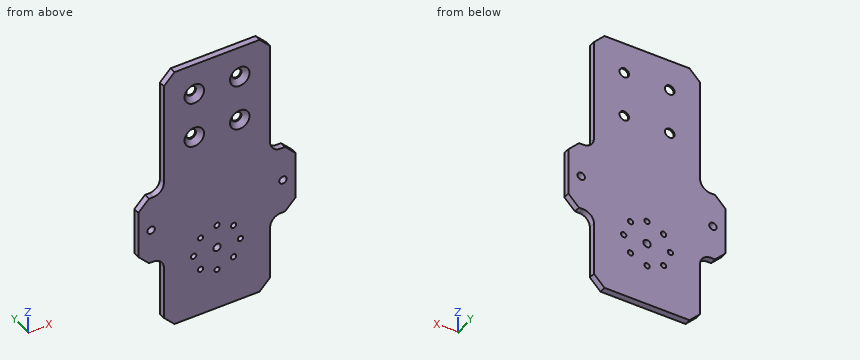
from build123d import *

# Parameters (mm, degrees)
SKETCH1_W                                    = 50
SKETCH1_H                                    = 125
BOSS_EXTRUDE1_DEPTH                          = 3
SKETCH2_R                                    = 1.75
CUT_EXTRUDE1_DEPTH                           = 10
SKETCH14_R                                   = 2
CUT_EXTRUDE16_DEPTH                          = 10
CSK_FOR_M4_HEX_SOCKET_COUNTERSUNK_HE_2_COUNT = 2
CSK_FOR_M4_HEX_SOCKET_COUNTERSUNK_HE_2_PITCH = 21.4
CSK_FOR_M4_HEX_SOCKET_COUNTERSUNK_HE_3_COUNT = 2
CSK_FOR_M4_HEX_SOCKET_COUNTERSUNK_HE_3_PITCH = 30.264170235
CSK_FOR_M4_HEX_SOCKET_COUNTERSUNK_HE_4_COUNT = 2
CSK_FOR_M4_HEX_SOCKET_COUNTERSUNK_HE_4_PITCH = 21.4
CUT_EXTRUDE17_REACH                          = 69.381
SKETCH18_R                                   = 1.25
CHAMFER1_SIZE                                = 5
SKETCH19_W                                   = 12
SKETCH19_H                                   = 32
BOSS_EXTRUDE2_DEPTH                          = 3
CHAMFER2_SIZE                                = 5
FILLET1_R                                    = 5
SKETCH20_R                                   = 1.75
CUT_EXTRUDE18_DEPTH                          = 73.692846966


with BuildPart() as part:
    # Sketch1 → Boss-Extrude1 (new body)
    with BuildSketch(Plane(origin=(0, 0, 0), x_dir=(1, 0, 0), z_dir=(0, 1, 0))):
        Rectangle(SKETCH1_W, SKETCH1_H)
    extrude(amount=BOSS_EXTRUDE1_DEPTH)

    # Sketch2 → Cut-Extrude1 (cut)
    with BuildSketch(Plane(origin=(0, 3, 0), x_dir=(1, 0, 0), z_dir=(0, 1, 0))):
        with Locations(Location((0, 32.5, 0), (0, 0, 270))):
            Circle(SKETCH2_R)
    extrude(amount=-CUT_EXTRUDE1_DEPTH, mode=Mode.SUBTRACT)

    # Sketch14 → Cut-Extrude16 (cut)
    with BuildSketch(Plane(origin=(0, 3, 0), x_dir=(1, 0, 0), z_dir=(0, 1, 0))):
        with Locations(Location((-10.7, -26.6, 0), (0, 0, 270))):
            Circle(SKETCH14_R)
        with Locations(Location((10.7, -26.6, 0), (0, 0, 270))):
            Circle(SKETCH14_R)
        with Locations(Location((10.7, -48, 0), (0, 0, 270))):
            Circle(SKETCH14_R)
        with Locations(Location((-10.7, -48, 0), (0, 0, 270))):
            Circle(SKETCH14_R)
    extrude(amount=-CUT_EXTRUDE16_DEPTH, mode=Mode.SUBTRACT)

    # Sketch15 → CSK for M4 Hex Socket Countersunk Head Screw1 (revolve, cut)
    with BuildSketch(Plane(origin=(-10.7, 0, 26.6), x_dir=(0, 0, -1), z_dir=(1, 0, 0))):
        Polygon((0, 0), (0, 3), (2.25, 3), (2.25, 2.34), (4.59, 0), align=None)
    csk_for_m4_hex_socket_countersunk_head_s = revolve(axis=Axis((-10.7, -6.35, 26.6), (0, 1, 0)), mode=Mode.SUBTRACT)

    # CSK for M4 Hex Socket Countersunk He 2: CSK for M4 Hex Socket Countersunk Head Screw1 ×2
    with Locations(*[(i * CSK_FOR_M4_HEX_SOCKET_COUNTERSUNK_HE_2_PITCH, 0, 0) for i in range(1, CSK_FOR_M4_HEX_SOCKET_COUNTERSUNK_HE_2_COUNT)]):
        add(csk_for_m4_hex_socket_countersunk_head_s, mode=Mode.SUBTRACT)

    # CSK for M4 Hex Socket Countersunk He 3: CSK for M4 Hex Socket Countersunk Head Screw1 ×2
    with Locations(*[Vector(0.7071067811865474, 0, 0.7071067811865477) * (i * CSK_FOR_M4_HEX_SOCKET_COUNTERSUNK_HE_3_PITCH) for i in range(1, CSK_FOR_M4_HEX_SOCKET_COUNTERSUNK_HE_3_COUNT)]):
        add(csk_for_m4_hex_socket_countersunk_head_s, mode=Mode.SUBTRACT)

    # CSK for M4 Hex Socket Countersunk He 4: CSK for M4 Hex Socket Countersunk Head Screw1 ×2
    with Locations(*[(0, 0, i * CSK_FOR_M4_HEX_SOCKET_COUNTERSUNK_HE_4_PITCH) for i in range(1, CSK_FOR_M4_HEX_SOCKET_COUNTERSUNK_HE_4_COUNT)]):
        add(csk_for_m4_hex_socket_countersunk_head_s, mode=Mode.SUBTRACT)

    # Sketch18 → Cut-Extrude17 (cut, up to next)
    with BuildSketch(Plane.XZ, mode=Mode.PRIVATE) as cut_extrude17_sk1:
        with Locations(Location((0, -21.5, 0), (0, 0, 270))):
            Circle(SKETCH18_R)
    cut_extrude17_tool1 = extrude(cut_extrude17_sk1.sketch, amount=-CUT_EXTRUDE17_REACH, mode=Mode.PRIVATE) & part.part
    # Sketch18 → Cut-Extrude17 (cut, up to next)
    with BuildSketch(Plane.XZ, mode=Mode.PRIVATE) as cut_extrude17_sk2:
        with Locations(Location((0, -43.5, 0), (0, 0, 270))):
            Circle(SKETCH18_R)
    cut_extrude17_tool2 = extrude(cut_extrude17_sk2.sketch, amount=-CUT_EXTRUDE17_REACH, mode=Mode.PRIVATE) & part.part
    # Sketch18 → Cut-Extrude17 (cut, up to next)
    with BuildSketch(Plane.XZ, mode=Mode.PRIVATE) as cut_extrude17_sk3:
        with Locations(Location((-11, -32.5, 0), (0, 0, 270))):
            Circle(SKETCH18_R)
    cut_extrude17_tool3 = extrude(cut_extrude17_sk3.sketch, amount=-CUT_EXTRUDE17_REACH, mode=Mode.PRIVATE) & part.part
    # Sketch18 → Cut-Extrude17 (cut, up to next)
    with BuildSketch(Plane.XZ, mode=Mode.PRIVATE) as cut_extrude17_sk4:
        with Locations(Location((11, -32.5, 0), (0, 0, 270))):
            Circle(SKETCH18_R)
    cut_extrude17_tool4 = extrude(cut_extrude17_sk4.sketch, amount=-CUT_EXTRUDE17_REACH, mode=Mode.PRIVATE) & part.part
    # Sketch18 → Cut-Extrude17 (cut, up to next)
    with BuildSketch(Plane.XZ, mode=Mode.PRIVATE) as cut_extrude17_sk5:
        with Locations(Location((7.778174593, -24.721825407, 0), (0, 0, 270))):
            Circle(SKETCH18_R)
    cut_extrude17_tool5 = extrude(cut_extrude17_sk5.sketch, amount=-CUT_EXTRUDE17_REACH, mode=Mode.PRIVATE) & part.part
    # Sketch18 → Cut-Extrude17 (cut, up to next)
    with BuildSketch(Plane.XZ, mode=Mode.PRIVATE) as cut_extrude17_sk6:
        with Locations(Location((-7.778174593, -24.721825407, 0), (0, 0, 270))):
            Circle(SKETCH18_R)
    cut_extrude17_tool6 = extrude(cut_extrude17_sk6.sketch, amount=-CUT_EXTRUDE17_REACH, mode=Mode.PRIVATE) & part.part
    # Sketch18 → Cut-Extrude17 (cut, up to next)
    with BuildSketch(Plane.XZ, mode=Mode.PRIVATE) as cut_extrude17_sk7:
        with Locations(Location((-7.778174593, -40.278174593, 0), (0, 0, 270))):
            Circle(SKETCH18_R)
    cut_extrude17_tool7 = extrude(cut_extrude17_sk7.sketch, amount=-CUT_EXTRUDE17_REACH, mode=Mode.PRIVATE) & part.part
    # Sketch18 → Cut-Extrude17 (cut, up to next)
    with BuildSketch(Plane.XZ, mode=Mode.PRIVATE) as cut_extrude17_sk8:
        with Locations(Location((7.778174593, -40.278174593, 0), (0, 0, 270))):
            Circle(SKETCH18_R)
    cut_extrude17_tool8 = extrude(cut_extrude17_sk8.sketch, amount=-CUT_EXTRUDE17_REACH, mode=Mode.PRIVATE) & part.part
    add(cut_extrude17_tool1.solids().sort_by_distance((0, 0, -21.5))[0], mode=Mode.SUBTRACT)
    add(cut_extrude17_tool2.solids().sort_by_distance((0, 0, -43.5))[0], mode=Mode.SUBTRACT)
    add(cut_extrude17_tool3.solids().sort_by_distance((-11, 0, -32.5))[0], mode=Mode.SUBTRACT)
    add(cut_extrude17_tool4.solids().sort_by_distance((11, 0, -32.5))[0], mode=Mode.SUBTRACT)
    add(cut_extrude17_tool5.solids().sort_by_distance((7.778175, 0, -24.721825))[0], mode=Mode.SUBTRACT)
    add(cut_extrude17_tool6.solids().sort_by_distance((-7.778175, 0, -24.721825))[0], mode=Mode.SUBTRACT)
    add(cut_extrude17_tool7.solids().sort_by_distance((-7.778175, 0, -40.278175))[0], mode=Mode.SUBTRACT)
    add(cut_extrude17_tool8.solids().sort_by_distance((7.778175, 0, -40.278175))[0], mode=Mode.SUBTRACT)

    # Chamfer1
    chamfer1_edges = [part.edges().sort_by_distance(p)[0] for p in [
        (-25, 1.5, -62.5),
        (25, 1.5, -62.5),
        (25, 1.5, 62.5),
        (-25, 1.5, 62.5),
    ]]
    chamfer(chamfer1_edges, length=CHAMFER1_SIZE)

    # Sketch19 → Boss-Extrude2 (add)
    with BuildSketch(Plane(origin=(0, 3, 0), x_dir=(1, 0, 0), z_dir=(0, 1, 0))):
        with Locations((-31, 11.5)):
            Rectangle(SKETCH19_W, SKETCH19_H)
        with Locations((31, 11.5)):
            Rectangle(SKETCH19_W, SKETCH19_H)
    extrude(amount=-BOSS_EXTRUDE2_DEPTH)

    # Chamfer2
    chamfer2_edges = [part.edges().sort_by_distance(p)[0] for p in [
        (37, 1.5, -27.5),
        (37, 1.5, 4.5),
        (-37, 1.5, -27.5),
        (-37, 1.5, 4.5),
    ]]
    chamfer(chamfer2_edges, length=CHAMFER2_SIZE)

    # Fillet1
    fillet1_edges = [part.edges().sort_by_distance(p)[0] for p in [
        (-25, 1.5, -27.5),
        (-25, 1.5, 4.5),
        (25, 1.5, -27.5),
        (25, 1.5, 4.5),
    ]]
    fillet(fillet1_edges, radius=FILLET1_R)

    # Sketch20 → Cut-Extrude18 (cut, through all)
    with BuildSketch(Plane(origin=(0, 3, 0), x_dir=(1, 0, 0), z_dir=(0, 1, 0))):
        with Locations(Location((-31, 11.5, 0), (0, 0, 270))):
            Circle(SKETCH20_R)
        with Locations(Location((31, 11.5, 0), (0, 0, 90))):
            Circle(SKETCH20_R)
    extrude(amount=-CUT_EXTRUDE18_DEPTH, mode=Mode.SUBTRACT)


solid = part.part
Check sheet for the modelled part. Datum: model origin and axes. Units: mm. Coordinates: 2 decimals unless noted, no trailing zeros. Write each loop counter-clockwise with the first axis right and the second up, starting at its lowest first coordinate (ties: lowest second). Pieces come first, ordered by that corner, then holes. Notation, with made-up numbers: M 56,74.5 L 115,74.5 A9 cw 115,87.5 Z; hole C 15,-16.75 d7. An arc over 180 degrees is marked long. Answer as CSV lines item,"result".
Q1. Cross-section at C-C (z = -43.5). Record the boundary of the cut face in (x, y).
Check result:
outline,"M -25,0 L -1.25,0 L -1.25,3 L -25,3 Z; M 1.25,0 L 25,0 L 25,3 L 1.25,3 Z"
Q2. Cross-section at D-D (y = 1.85). Count the separate pieces of the cut face and the enclosed holes in it, then the cut area to 3 significant figures.
Check result:
separate pieces,"1"
enclosed holes,"15"
area,"6,780 mm^2"
Q3. Material ranges on probe 1 along X at (y, z) = (2.8, 48); probe 2 along X at (y, z) = (0.25, -24); probe 3 along X at (y, z) = (1.65, -43.5), recorded low to high. Write a range as from..to.
Check result:
probe 1,"-25..-12.95, -8.45..8.45, 12.95..25"
probe 2,"-35.5..-8.8, -6.76..6.76, 8.8..35.5"
probe 3,"-25..-1.25, 1.25..25"
Q4. Cross-section at B-B (x = 0). Record the boundary of the cut face in (y, z).
Check result:
outline,"M 0,-62.5 L 3,-62.5 L 3,-44.75 L 0,-44.75 Z; M 0,-42.25 L 3,-42.25 L 3,-34.25 L 0,-34.25 Z; M 0,-30.75 L 3,-30.75 L 3,-22.75 L 0,-22.75 Z; M 0,-20.25 L 3,-20.25 L 3,62.5 L 0,62.5 Z"
Q5. Cross-section at A-A (z = -11.5). Record the boundary of the cut face in (x, y).
Check result:
outline,"M -37,0 L -32.75,0 L -32.75,3 L -37,3 Z; M -29.25,0 L 29.25,0 L 29.25,3 L -29.25,3 Z; M 32.75,0 L 37,0 L 37,3 L 32.75,3 Z"
Q6. Go/stop test with flat-tipped pins: pin 1 (6 mm diameter, centred on x = -10.7, z = 48, fed in from -Y); pin 2 (1.5 mm diameter, centred on x = 0, z = -43.5, fed in from -Y); pin 3 (0.6 mm diameter, centred on x = 31.5, y = 1, fed in from -Z); pin 4 (1.5 mm diameter, centred on y = 1.5, z = -45, fed in from -X). Record where each tip stops, or that it passes through.
Check result:
pin 1,"y = 1.59"
pin 2,"through"
pin 3,"z = -27.5"
pin 4,"x = -25"
